Part model, mm, in its own coordinate system. Face numbers are marked on the shaded views. A direction names the side the tool comes from. Give positions to 0.01 mm unless a question says otherwise; leave off trailing zeros. Order: outer loops, then holes, each group sorted by start corner. A loop starts at its lowest first (then second) coordinate and runs counter-clockwise, first axis right, second up. Notation, with made-up numbers: (-8, -33) - (31, -33) arc R25 ccw to (31, 0) - close; hole circle Ø2 at (48, 62.25). An arc over 180 degrees is marked (long way). One line per item, written item: value.
```python
from build123d import *

# Parameters (mm, degrees)
F1_DEPTH = 105
F2_W     = 40
F2_H     = 10
F3_DEPTH = 25
F5_DEPTH = 25
F7_D     = 5
F8_R     = 2
F9_R     = 2


with BuildPart() as f1:
    # F0 (on Right) → F1 (new body)
    with BuildSketch(Plane.YZ):
        Polygon((0, 38), (0, 0), (6, 0), (6, 32), (38, 32), (38, 38), align=None)
    extrude(amount=F1_DEPTH)

    # F2 (on face) → F3 (cut)
    with BuildSketch(Plane.XZ):
        with Locations((85, 5)):
            Rectangle(F2_W, F2_H)
    extrude(amount=-F3_DEPTH, mode=Mode.SUBTRACT)

    # F4 (on face) → F5 (cut)
    with BuildSketch(Plane(origin=(0, 6, 0), x_dir=(-1, 0, 0), z_dir=(0, 1, 0))):
        with BuildLine():
            ThreePointArc((-97, 14.7), (-94.6665476221, 15.6665476221), (-93.7, 18))
            ThreePointArc((-93.7, 18), (-94.6665476221, 20.3334523779), (-97, 21.3))
            ThreePointArc((-97, 21.3), (-100.3, 18), (-97, 14.7))
        make_face()
        with BuildLine():
            ThreePointArc((-97, 21.3), (-94.6665476221, 20.3334523779), (-93.7, 18))
            ThreePointArc((-93.7, 18), (-94.6665476221, 15.6665476221), (-97, 14.7))
            Line((-97, 14.7), (-83, 14.7))
            ThreePointArc((-83, 14.7), (-86.3, 18), (-83, 21.3))
            Line((-83, 21.3), (-97, 21.3))
        make_face()
        with BuildLine():
            Line((-83, 14.7), (-83, 21.3))
            ThreePointArc((-83, 21.3), (-86.3, 18), (-83, 14.7))
        make_face()
        with BuildLine():
            ThreePointArc((-79.7, 18), (-80.6665476221, 20.3334523779), (-83, 21.3))
            Line((-83, 21.3), (-83, 14.7))
            ThreePointArc((-83, 14.7), (-80.6665476221, 15.6665476221), (-79.7, 18))
        make_face()
        with BuildLine():
            ThreePointArc((-52, 14.7), (-49.6665476221, 15.6665476221), (-48.7, 18))
            ThreePointArc((-48.7, 18), (-49.6665476221, 20.3334523779), (-52, 21.3))
            ThreePointArc((-52, 21.3), (-55.3, 18), (-52, 14.7))
        make_face()
        with BuildLine():
            ThreePointArc((-52, 21.3), (-49.6665476221, 20.3334523779), (-48.7, 18))
            ThreePointArc((-48.7, 18), (-49.6665476221, 15.6665476221), (-52, 14.7))
            Line((-52, 14.7), (-38, 14.7))
            ThreePointArc((-38, 14.7), (-41.3, 18), (-38, 21.3))
            Line((-38, 21.3), (-52, 21.3))
        make_face()
        with BuildLine():
            Line((-38, 14.7), (-38, 21.3))
            ThreePointArc((-38, 21.3), (-41.3, 18), (-38, 14.7))
        make_face()
        with BuildLine():
            ThreePointArc((-34.7, 18), (-35.6665476221, 20.3334523779), (-38, 21.3))
            Line((-38, 21.3), (-38, 14.7))
            ThreePointArc((-38, 14.7), (-35.6665476221, 15.6665476221), (-34.7, 18))
        make_face()
    extrude(amount=-F5_DEPTH, mode=Mode.SUBTRACT)

    # F7 (through all)
    with Locations(Plane.XY.offset(38)):
        with Locations((31, 18), (17, 26)):
            Hole(F7_D / 2)

    # F8
    f8_edges = [f1.edges().sort_by_distance(p)[0] for p in [
        (52.5, 38, 32),
        (32.5, 6, 0),
    ]]
    fillet(f8_edges, radius=F8_R)

    # F9
    f9_edges = [f1.edges().sort_by_distance(p)[0] for p in [
        (52.5, 6, 32),
    ]]
    fillet(f9_edges, radius=F9_R)


solid = f1.part
```
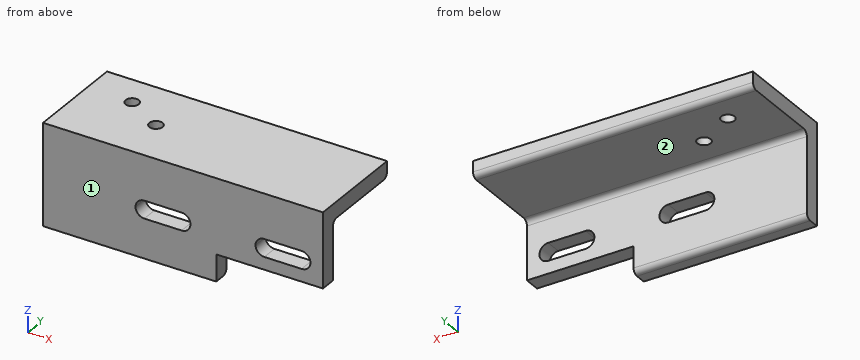
1) Cut at A-A, the plane y = 26. Give the cut face in (x, z), then the cut area to 3 significant figures.
Outcome:
outline: (0, 32) - (14.5, 32) - (14.5, 38) - (0, 38) - close; (19.5, 32) - (105, 32) - (105, 38) - (19.5, 38) - close
area: 600 mm^2
2) Drill centre lines: line 1 along Y through (x, z) = (31, 34.85); line 2 along Z through (x, y) = (17, 17.5); line 3 along Y through (x, z) = (60.5, 6.5). Where is each one in solid material? Low to high. Write a range as from..to.
Outcome:
line 1: y = 0..15.5, 20.5..38
line 2: z = 32..38
line 3: y = 0..6
3) Pin check, flat tips, straight feed: pin 1 (8.5 mm diameter, centred on x = 37.5, z = 16.5, fed in from +Y); pin 2 (1.8 mm diameter, centred on y = 2.5, z = 6.5, fed in from +X); pin 3 (4 mm diameter, centred on x = 13.5, y = 11.5, fed in from -Z). Stop position of each tip, or through.
Outcome:
pin 1: stops at y = 6
pin 2: stops at x = 65
pin 3: stops at z = 32
4) Cut at B-B, the plane x = 40.5. Give the cut face in (y, z).
Outcome:
outline: (0, 0) - (4, 0) arc R2 ccw to (6, 2) - (6, 14.7) - (0, 14.7) - close; (0, 21.3) - (6, 21.3) - (6, 30) arc R2 cw to (8, 32) - (36, 32) arc R2 ccw to (38, 34) - (38, 38) - (0, 38) - close
5) Cut at C-C, the plane z = 19. Give the cut face in (x, y).
Outcome:
outline: (0, 0) - (34.86, 0) - (34.86, 6) - (0, 6) - close; (55.14, 0) - (79.86, 0) - (79.86, 6) - (55.14, 6) - close; (100.14, 0) - (105, 0) - (105, 6) - (100.14, 6) - close
6) Which spindle directions (+Z, -Z, +X, -X, +Y, -Y) get a long thin tool onto all of the face, cutting with end or side? Do the marked faces 1 and 2. Say none if no direction does.
Outcome:
face 1: +Z, -Z, +X, -X, -Y
face 2: -Z, +X, -X, +Y
7) Cut at D-D, the plane x = 25. Give the cut face in (y, z), then the cut area to 3 significant figures.
Outcome:
outline: (0, 0) - (4, 0) arc R2 ccw to (6, 2) - (6, 30) arc R2 cw to (8, 32) - (36, 32) arc R2 ccw to (38, 34) - (38, 38) - (0, 38) - close
area: 419 mm^2
